Model file for the job. Use its own axes, mm. Face numbers are marked on the shaded views. Round coordinates to 2 decimals unless told otherwise and drop trailing zeros. Order: outer loops, then holes, each group sorted by start corner. A loop starts at its lowest first (then second) coordinate and runs counter-clockwise, first axis right, second up. Notation, with made-up numbers: M 24,80 L 72,80 A30 ccw 72,105 Z; hole C 74,28 d11. An arc over 180 degrees is marked long. Return JSON: item names as keys, results as strings. Group by question number.
Item 1: Slice it at B-B on x = 42.25. Write the cut outline in (y, z), then the cut area to 3 significant figures.
Item 2: Probe line 1 along Z through (x, y) = (1, -2.6); line 2 along X through (y, z) = (-1.2, -3.75); line 3 along Y through (x, z) = (-31.5, -4). List the from-to ranges inside material, lowest first.
Item 3: Slice it at D-D on z = -5.5. Write the cut outline in (x, y).
Item 4: Pin check, flat tip, straight feed: pin 1 Ø3 at (x, z) = (28.5, -1.5) entering from +Y. Stop position of the tip, or through.
Item 5: Slice it at C-C on z = 0. Write the cut outline in (x, y), then the cut area to 3 significant figures.
Item 6: Slice it at A-A on y = -0.6. Write the cut outline in (x, z).
Item 7: Pull direction X, two halves, no side cores. Call the marked faces 1 and 2: pulls with the +X half, pulls with the -X half, needs draft (parallel to the pull), parting line crosses it, or undercut.
from build123d import *

# Parameters (mm, degrees)
F0_W      = 100
F0_H      = 15
F0_W_2    = 63
F0_H_2    = 3
F1_DEPTH  = 4
F2_W      = 69
F2_H      = 15
F3_DEPTH  = 2
F4_R      = 2.5
F5_DEPTH  = 25
F6_R      = 2.5
F7_DEPTH  = 25
F8_W      = 9
F8_H      = 3
F9_DEPTH  = 2
F10_R     = 1.5
F11_DEPTH = 25
F12_W     = 68.882376
F12_H     = 7.5
F13_DEPTH = 2


with BuildPart() as f1:
    # F0 (on Front) → F1 (new body)
    with BuildSketch(Plane.XZ):
        Rectangle(F0_W, F0_H)
        with Locations((0, -3)):
            Rectangle(F0_W_2, F0_H_2, mode=Mode.SUBTRACT)
        with Locations((0, 3)):
            Rectangle(F0_W_2, F0_H_2, mode=Mode.SUBTRACT)
    extrude(amount=F1_DEPTH)

    # F2 (on face) → F3 (cut)
    with BuildSketch(Plane(origin=(0, 0, 0), x_dir=(-1, 0, 0), z_dir=(0, 1, 0))):
        Rectangle(F2_W, F2_H)
    extrude(amount=-F3_DEPTH, mode=Mode.SUBTRACT)

    # F4 (on face) → F5 (cut)
    with BuildSketch(Plane(origin=(0, 0, 0), x_dir=(-1, 0, 0), z_dir=(0, 1, 0))):
        with Locations((-42.25, 0)):
            Circle(F4_R)
    extrude(amount=-F5_DEPTH, mode=Mode.SUBTRACT)

    # F6 (on face) → F7 (cut)
    with BuildSketch(Plane(origin=(0, 0, 0), x_dir=(-1, 0, 0), z_dir=(0, 1, 0))):
        with Locations((42.25, 0)):
            Circle(F6_R)
    extrude(amount=-F7_DEPTH, mode=Mode.SUBTRACT)

    # F8 (on face) → F9 (join)
    with BuildSketch(Plane.XZ.offset(4)):
        with Locations((27, 3)):
            Rectangle(F8_W, F8_H)
    extrude(amount=-F9_DEPTH)

    # F10 (on face) → F11 (cut)
    with BuildSketch(Plane.XZ.offset(4)):
        with Locations((27, 3)):
            Circle(F10_R)
    extrude(amount=-F11_DEPTH, mode=Mode.SUBTRACT)

    # F12 (on face) → F13 (join)
    with BuildSketch(Plane.XZ.offset(4)):
        with Locations((0.509296, -3.75)):
            Rectangle(F12_W, F12_H)
    extrude(amount=-F13_DEPTH)


solid = f1.part
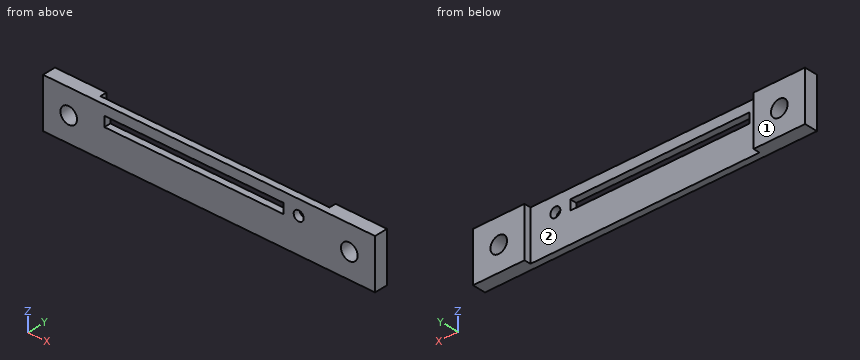
Output values:
{
 "1": {"outline": "M -4,-7.5 L 0,-7.5 L 0,-2.5 L -4,-2.5 Z; M -4,2.5 L 0,2.5 L 0,7.5 L -4,7.5 Z", "area": "40.0 mm²"},
 "2": {"line 1": "-7.5 to 1.5, 4.5 to 7.5", "line 2": "-50 to -34.5, 34.5 to 50", "line 3": "-4 to -2"},
 "3": {"outline": "M -50,-4 L 50,-4 L 50,0 L 34.5,0 L 34.5,-2 L -34.5,-2 L -34.5,0 L -50,0 Z"},
 "4": {"pin 1": "y = -2"},
 "5": {"outline": "M -50,-4 L -44.75,-4 L -44.75,0 L -50,0 Z; M -39.75,-4 L 39.75,-4 L 39.75,0 L 34.5,0 L 34.5,-2 L -34.5,-2 L -34.5,0 L -39.75,0 Z; M 44.75,-4 L 50,-4 L 50,0 L 44.75,0 Z", "area": "222 mm²"},
 "6": {"outline": "M -50,-7.5 L -34.5,-7.5 L -34.5,7.5 L -50,7.5 Z; M 34.5,-7.5 L 50,-7.5 L 50,7.5 L 34.5,7.5 Z; hole C -42.25,0 d5; hole C 42.25,0 d5"},
 "7": {"face 1": "needs draft", "face 2": "undercut"}
}
